Geometry: final body of the model. Coordinates: model frame, mm. Face numbers are marked on the shaded views. Give positions to 0.01 mm unless a question says otherwise; leave off trailing zeros. Loops run counter-clockwise (first coordinate to the right, second up) from the corner with the lowest first, then second, coordinate; pieces in that order, holes last.
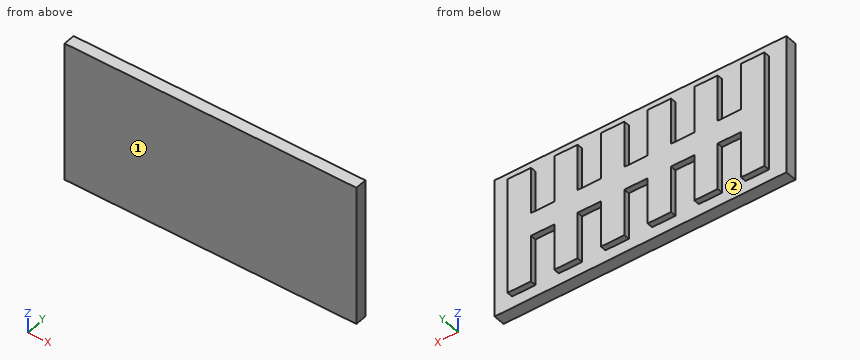
```python
from build123d import *

# Parameters (mm, degrees)
SKETCH1_W           = 25
SKETCH1_H           = 12
BOSS_EXTRUDE1_DEPTH = 1
WRAP1_DEPTH         = 0.5


# Read off the part's stored shape, not the designer's step: Wrap1
with BuildPart() as part:
    # Sketch1 → Boss-Extrude1 (new body)
    with BuildSketch(Plane(origin=(0, 0, 0), x_dir=(1, 0, 0), z_dir=(0, 1, 0))):
        Rectangle(SKETCH1_W, SKETCH1_H)
    extrude(amount=BOSS_EXTRUDE1_DEPTH)

    # Wrap1 outline → Wrap1 (add)
    with BuildSketch(Plane(origin=(0, 1, 0), x_dir=(1, 0, 0), z_dir=(0, 1, 0))):
        Polygon((-11, -5), (-9, -5), (-9, -1), (-7, -1), (-7, -5), (-5, -5), (-5, -1), (-3, -1), (-3, -5), (-1, -5), (-1, -1), (1, -1), (1, -5), (3, -5), (3, -1), (5, -1), (5, -5), (7, -5), (7, -1), (9, -1), (9, -5), (11, -5), (11, 5), (9, 5), (9, 1), (7, 1), (7, 5), (5, 5), (5, 1), (3, 1), (3, 5), (1, 5), (1, 1), (-1, 1), (-1, 5), (-3, 5), (-3, 1), (-5, 1), (-5, 5), (-7, 5), (-7, 1), (-9, 1), (-9, 5), (-11, 5), align=None)
    extrude(amount=WRAP1_DEPTH)


solid = part.part
```
Q1. Mould query, pull axis X, two halves, no side actions, for the marked faces 1 and 2. Classes: +X half, -X half, draft (parallel to the pull), parting line (faces both ways), or undercut.
Q2. Pin query (flat end, axial travel): pin 1 Ø0.6 at (y, z) = (1.5, 3) entering from -X; pin 2 Ø0.6 at (y, z) = (1.5, -2.5) entering from +X. Return the tip coordinate at first contact, or that it passes through.
Q3. Section query A-A, the plane z = 3. Return loops of the section in (x, y).
Q4. Material intervals for probe 1 along X at (y, z) = (1.4, -1.5); probe 2 along Y at (x, z) = (6, 5.5); probe 3 along X at (y, z) = (1.35, -0.25), sorted ascending.
Q5. Section query B-B, the plane x = -8.5. Return loops of the section in (y, z).
Q6. Section query C-C, the plane x = 2. Return loops of the section in (y, z), and give its area (3 significant figures).
Resolved:
1. face 1: draft
1. face 2: undercut
2. pin 1: stops at x = -11
2. pin 2: stops at x = 11
3. outline: (-12.5, 0) - (12.5, 0) - (12.5, 1) - (11, 1) - (11, 1.5) - (9, 1.5) - (9, 1) - (7, 1) - (7, 1.5) - (5, 1.5) - (5, 1) - (3, 1) - (3, 1.5) - (1, 1.5) - (1, 1) - (-1, 1) - (-1, 1.5) - (-3, 1.5) - (-3, 1) - (-5, 1) - (-5, 1.5) - (-7, 1.5) - (-7, 1) - (-9, 1) - (-9, 1.5) - (-11, 1.5) - (-11, 1) - (-12.5, 1) - close
4. probe 1: x = -11 to -9, -7 to -5, -3 to -1, 1 to 3, 5 to 7, 9 to 11
4. probe 2: y = 0 to 1
4. probe 3: x = -11 to 11
5. outline: (0, -6) - (1, -6) - (1, -1) - (1.5, -1) - (1.5, 1) - (1, 1) - (1, 6) - (0, 6) - close
6. outline: (0, -6) - (1, -6) - (1, -5) - (1.5, -5) - (1.5, 5) - (1, 5) - (1, 6) - (0, 6) - close
6. area: 17.0 mm2
